Check sheet for the modelled part. Datum: model origin and axes. Units: mm. Round coordinates to 2 decimals unless told otherwise and drop trailing zeros. Order: outer loops, then holes, each group sorted by start corner. A loop starts at its lowest first (then second) coordinate and runs counter-clockwise, first axis right, second up.
from build123d import *

# Parameters (mm, degrees)
SKETCH1_R           = 4.9625
BOSS_EXTRUDE1_DEPTH = 4.37
FILLET1_R           = 5
SKETCH2_R           = 1.65
CUT_EXTRUDE1_DEPTH  = 5.37


with BuildPart() as part:
    # Sketch1 → Boss-Extrude1 (new body)
    with BuildSketch(Plane(origin=(0, 0, 0), x_dir=(0, 0, -1), z_dir=(1, 0, 0))):
        with BuildLine():
            Line((0, 7.5), (12, 7.5))
            Line((12, 7.5), (12, -7.5))
            Line((12, -7.5), (0, -7.5))
            ThreePointArc((0, -7.5), (-7.5, 0), (0, 7.5))
        make_face()
        Circle(SKETCH1_R, mode=Mode.SUBTRACT)
    extrude(amount=BOSS_EXTRUDE1_DEPTH)

    # Fillet1
    fillet1_edges = [part.edges().sort_by_distance(p)[0] for p in [
        (2.185, -7.5, -12),
        (2.185, 7.5, -12),
    ]]
    fillet(fillet1_edges, radius=FILLET1_R)

    # Sketch2 → Cut-Extrude1 (cut, through all)
    with BuildSketch(Plane.ZY):
        with Locations((-6.905099565, 4)):
            Circle(SKETCH2_R)
        with Locations((-6.905099565, -4)):
            Circle(SKETCH2_R)
    extrude(amount=-CUT_EXTRUDE1_DEPTH, mode=Mode.SUBTRACT)


solid = part.part
1) Gauge pin test, flat end, axial feed: pin 1 (5.5 mm diameter, centred on y = 4, z = -6.91, fed in from +X). Record the tip position at first contact, or that the pin passes through.
2) Sectioned sample at D-D on y = 3. Record the cut outline in (x, z).
3) Scan lines: line 1 (Y direction, x = 3.3, z = -7.5); line 2 (Z direction, x = 1.35, y = -2.5); line 3 (Y direction, x = 4.1, z = 1). Record each from-to range of solid material in increasing order.
4) Sectioned sample at B-B on z = 0.75. Record the cut outline in (x, y).
5) Sectioned sample at A-A on y = 0. Record the cut outline in (x, z).
6) Draft check along Y on faces 1 (the face through (2.154, -3.927, -8.554)), 2 (the face through (2.15, -0.16, 7.5)), 3 (the face through (0, 0, -7)). Enter one of: pulls with the +Y half, pulls with the -Y half, needs draft (parallel to the pull), parting line crosses it, or undercut.
7) Sectioned sample at C-C on y = -4.75. Record the cut outline in (x, z), and give its area (3 significant figures).
Values found:
1. pin 1: stops at x = 4.37
2. outline: (0, -11.97) - (4.37, -11.97) - (4.37, -8.22) - (0, -8.22) - close; (0, -5.59) - (4.37, -5.59) - (4.37, -3.95) - (0, -3.95) - close; (0, 3.95) - (4.37, 3.95) - (4.37, 6.87) - (0, 6.87) - close
3. line 1: y = -7.47 to -5.54, -2.46 to 2.46, 5.54 to 7.47
3. line 2: z = -12 to -7.59, -6.22 to -4.29, 4.29 to 7.07
3. line 3: y = -7.43 to -4.86, 4.86 to 7.43
4. outline: (0, -7.46) - (4.37, -7.46) - (4.37, -4.91) - (0, -4.91) - close; (0, 4.91) - (4.37, 4.91) - (4.37, 7.46) - (0, 7.46) - close
5. outline: (0, -12) - (4.37, -12) - (4.37, -4.96) - (0, -4.96) - close; (0, 4.96) - (4.37, 4.96) - (4.37, 7.5) - (0, 7.5) - close
6. face 1: undercut
6. face 2: parting line crosses it
6. face 3: needs draft
7. outline: (0, -11.47) - (4.37, -11.47) - (4.37, -8.37) - (0, -8.37) - close; (0, -5.44) - (4.37, -5.44) - (4.37, -1.44) - (0, -1.44) - close; (0, 1.44) - (4.37, 1.44) - (4.37, 5.8) - (0, 5.8) - close
7. area: 50.1 mm2
